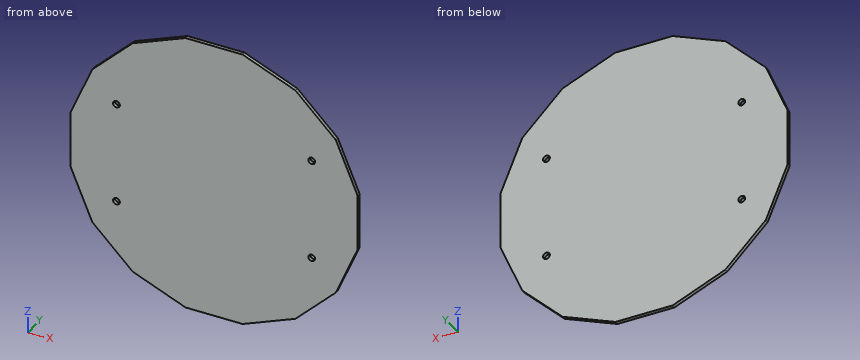
```python
from build123d import *

# Parameters (mm, degrees)
BOSS_EXTRUDE1_DEPTH = 1.6
SKETCH6_R           = 1.5
CUT_EXTRUDE2_DEPTH  = 1.6


with BuildPart() as part:
    # Sketch1 → Boss-Extrude1 (new body)
    with BuildSketch(Plane(origin=(0, 0, 0), x_dir=(1, 0, 0), z_dir=(0, 1, 0))):
        Polygon((62.5, 12.432022961), (52.984941564, 35.403406084), (35.403406084, 52.984941564), (12.432022961, 62.5), (-12.432022961, 62.5), (-35.403406084, 52.984941564), (-52.984941564, 35.403406084), (-62.5, 12.432022961), (-62.5, -12.432022961), (-52.984941564, -35.403406084), (-35.403406084, -52.984941564), (-12.432022961, -62.5), (12.432022961, -62.5), (35.403406084, -52.984941564), (52.984941564, -35.403406084), (62.5, -12.432022961), align=None)
    extrude(amount=BOSS_EXTRUDE1_DEPTH)

    # Sketch6 → Cut-Extrude2 (cut)
    with BuildSketch(Plane(origin=(0, 1.6, 0), x_dir=(1, 0, 0), z_dir=(0, 1, 0))):
        with Locations(Location((-42.5, 22.5, 0), (0, 0, 270))):
            Circle(SKETCH6_R)
        with Locations(Location((-42.5, -22.5, 0), (0, 0, 270))):
            Circle(SKETCH6_R)
        with Locations(Location((42.5, -22.5, 0), (0, 0, 270))):
            Circle(SKETCH6_R)
        with Locations(Location((42.5, 22.5, 0), (0, 0, 270))):
            Circle(SKETCH6_R)
    extrude(amount=-CUT_EXTRUDE2_DEPTH, mode=Mode.SUBTRACT)


solid = part.part
```
CAD build for the part. Positions are in the model's coordinates, mm. Round coordinates to 2 decimals unless told otherwise and drop trailing zeros. Write each loop counter-clockwise with the first axis right and the second up, starting at its lowest first coordinate (ties: lowest second). Pieces come first, ordered by that corner, then holes. Notation, with made-up numbers: M 12.5,24.25 L 38.5,24.25 A9 cw 38.5,36.25 Z; hole C -14.75,85 d11. An arc over 180 degrees is marked long. One line per question, with ' | ' between items.
1. Cut at A-A on y = 1. Write the cut outline in (x, z).
Working result:
outline: M -62.5,-12.43 L -52.98,-35.4 L -35.4,-52.98 L -12.43,-62.5 L 12.43,-62.5 L 35.4,-52.98 L 52.98,-35.4 L 62.5,-12.43 L 62.5,12.43 L 52.98,35.4 L 35.4,52.98 L 12.43,62.5 L -12.43,62.5 L -35.4,52.98 L -52.98,35.4 L -62.5,12.43 Z; hole C -42.5,-22.5 d3; hole C -42.5,22.5 d3; hole C 42.5,-22.5 d3; hole C 42.5,22.5 d3
2. Cut at B-B on x = 42.5. Write the cut outline in (y, z), and give its area (3 significant figures).
Working result:
outline: M 0,-45.89 L 1.6,-45.89 L 1.6,-24 L 0,-24 Z; M 0,-21 L 1.6,-21 L 1.6,21 L 0,21 Z; M 0,24 L 1.6,24 L 1.6,45.89 L 0,45.89 Z | area: 137 mm2
3. Cut at C-C on z = 22.5. Write the cut outline in (x, y), and give its area (3 significant figures).
Working result:
outline: M -58.33,0 L -44,0 L -44,1.6 L -58.33,1.6 Z; M -41,0 L 41,0 L 41,1.6 L -41,1.6 Z; M 44,0 L 58.33,0 L 58.33,1.6 L 44,1.6 Z | area: 177 mm2
4. Probe L1, parallel to X at y = 0.6, z = 23; L2, parallel to X at y = 1.25, z = -22.5; L3, parallel to Z at x = 21.5, y = 1.05. List the from-to ranges inside material, lowest first. Write a range as from..to.
Working result:
L1: -58.12..-43.91, -41.09..41.09, 43.91..58.12 | L2: -58.33..-44, -41..41, 44..58.33 | L3: -58.74..58.74
5. Cut at D-D on z = -17.5. Write the cut outline in (x, y).
Working result:
outline: M -60.4,0 L 60.4,0 L 60.4,1.6 L -60.4,1.6 Z
